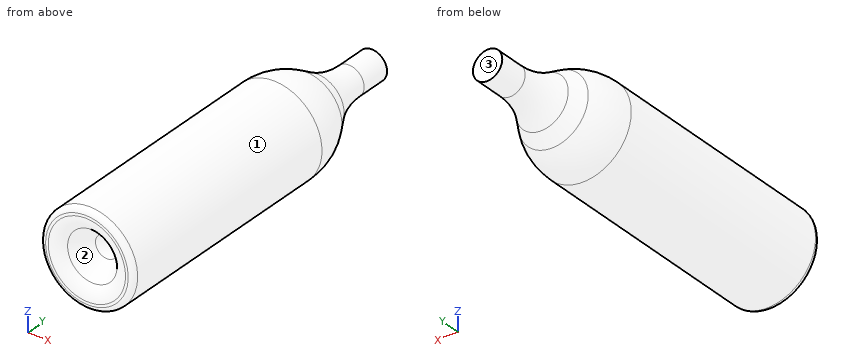
```python
from build123d import *


with BuildPart() as part:
    # Sketch2 → Revolve1 (revolve)
    with BuildSketch(Plane.XY):
        with BuildLine():
            Line((0, 274), (-11, 274))
            Line((-11, 274), (-11, 252))
            ThreePointArc((-11, 252), (-13.208083332, 236.288670718), (-19.661258519, 221.794601939))
            Line((-19.661258519, 221.794601939), (-26.338741481, 211.108395388))
            ThreePointArc((-26.338741481, 211.108395388), (-32.791916668, 196.614326608), (-35, 180.902997327))
            Line((-35, 180.902997327), (-35, 4))
            ThreePointArc((-35, 4), (-33.828427125, 1.171572875), (-31, 0))
            Line((-31, 0), (-29, 0))
            ThreePointArc((-29, 0), (-23.169165423, 1.380991086), (-18.577150935, 5.230558749))
            Line((-18.577150935, 5.230558749), (-8.361917252, 18.934483574))
            ThreePointArc((-8.361917252, 18.934483574), (-4.536719094, 21.540170522), (0, 22.456644901))
            Line((0, 22.456644901), (0, 274))
        make_face()
    revolve(axis=Axis((0, 0, 0), (0, 1, 0)))


solid = part.part
```
Check sheet for the modelled part. Datum: model origin and axes. Units: mm. Face numbers are marked on the shaded views. Give positions to 0.01 mm unless a question says otherwise; leave off trailing zeros. Write each loop counter-clockwise with the first axis right and the second up, starting at its lowest first coordinate (ties: lowest second). Pieces come first, ordered by that corner, then holes.
Item 1: Draft check along Z on the marked faces 1, 2 and 3. Enter one of: released by +Z, released by -Z, zero draft, split by the parting line, or undercut.
Item 2: Cross-section at A-A (y = 124). Enter the section's corners in (x, z), and give its area (3 significant figures).
Item 3: Scan lines: L1, parallel to X at y = 236.5, z = 4; L2, parallel to Y at x = -28.5, z = -1; L3, parallel to Y at x = 14, z = -15. Record each from-to range of solid material in increasing order.
Item 4: Gauge pin test, flat ends, axial feed: pin 1 (5 mm diameter, centred on y = 174, z = -12.5, fed in from +X); pin 2 (4 mm diameter, centred on y = 187, z = 9.5, fed in from +X); pin 3 (4 mm diameter, centred on y = 175.5, z = 9, fed in from +X). Record the tip position at first contact, or that the pin passes through.
Report:
1. face 1: split by the parting line
1. face 2: undercut
1. face 3: zero draft
2. outline: circle Ø70 at (0, 0)
2. area: 3,850 mm2
3. L1: x = -12.52 to 12.52
3. L2: y = 0.01 to 207.3
3. L3: y = 3.15 to 220.42
4. pin 1: stops at x = 33.54
4. pin 2: stops at x = 33.9
4. pin 3: stops at x = 34.29
